```python
from build123d import *

# Parameters (mm, degrees)
BOSS_EXTRUDE1_DEPTH     = 11.5
SKETCH2_R               = 1.5
CUT_EXTRUDE1_DEPTH      = 1
CUT_EXTRUDE1_DEPTH_BACK = 15.4
FILLET1_R               = 1
FILLET2_R               = 1
FILLET3_R               = 1


with BuildPart() as part:
    # Sketch1 → Boss-Extrude1 (new body, symmetric)
    with BuildSketch(Plane.XY):
        Polygon((-5.2, 1), (5.2, 1), (5.2, 13.5), (7.2, 13.5), (7.2, -1), (-7.2, -1), (-7.2, 13.5), (-5.2, 13.5), align=None)
    extrude(amount=BOSS_EXTRUDE1_DEPTH, both=True)

    # Sketch2 → Cut-Extrude1 (cut, two sides)
    with BuildSketch(Plane(origin=(7.2, 0, 0), x_dir=(0, 0, -1), z_dir=(1, 0, 0))) as cut_extrude1_sk:
        with Locations((-7, 9)):
            Circle(SKETCH2_R)
        with Locations((7, 9)):
            Circle(SKETCH2_R)
    extrude(amount=CUT_EXTRUDE1_DEPTH, mode=Mode.SUBTRACT)
    extrude(cut_extrude1_sk.sketch, amount=-CUT_EXTRUDE1_DEPTH_BACK, mode=Mode.SUBTRACT)

    # Fillet1
    fillet1_edges = [part.edges().sort_by_distance(p)[0] for p in [
        (0, -1, -11.5),
        (0, -1, 11.5),
    ]]
    fillet(fillet1_edges, radius=FILLET1_R)

    # Fillet2
    fillet2_edges = [part.edges().sort_by_distance(p)[0] for p in [
        (-5.2, 1, 0),
        (5.2, 1, 0),
    ]]
    fillet(fillet2_edges, radius=FILLET2_R)

    # Fillet3
    fillet3_edges = [part.edges().sort_by_distance(p)[0] for p in [
        (-6.2, 13.5, -11.5),
        (6.2, 13.5, 11.5),
        (-6.2, 13.5, 11.5),
        (6.2, 13.5, -11.5),
    ]]
    fillet(fillet3_edges, radius=FILLET3_R)


solid = part.part
```
CAD build for the part. Positions are in the model's coordinates, mm. Coordinates: 2 decimals unless noted, no trailing zeros. Loops run counter-clockwise (first coordinate to the right, second up) from the corner with the lowest first, then second, coordinate; pieces in that order, holes last. Notation, with made-up numbers: (0, 48) - (29, 48) arc R10 cw to (29, 56) - close; hole circle Ø1 at (-33.5, -0.5). An arc over 180 degrees is marked (long way). Use CSV: the item, a comma, the result in double quotes. Start each with the question number.
Q1. Probe probe 1 along X at (y, z) = (9.5, 4); probe 2 along Y at (x, z) = (6.45, -7); probe 3 along Y at (x, z) = (-2, -6.5). List the from-to ranges inside material, lowest first. Write a range as from..to.
Q2. Two-plate mould, pull along X, no slides. Class faces 1 (the cylindrical face through (-0.101, -0.699, -11.215)), 2 (the flat face through (0, 1, 0)), 3 (the flat face through (7.2, 6, 0)), 4 (the cylindrical face through (4.915, 1.301, -0.161)): +X half, -X half, draft (parallel to the pull), parting line (faces both ways), or undercut.
Q3. Drop flat-ended pins along their axis: P1, Ø2, axis at x = -2, z = -9, coming from the +Y side; P2, Ø2.5, axis at y = 9, z = -7, coming from the -X side. Give the stop position or say it passes through.
Q4. Cut at B-B, the plane z = -7. List the corners of the cut face in (x, y).
Q5. Cut at A-A, the plane y = 9. List the corners of the cut face in (x, z), then the cut area to 3 significant figures.
Q6. Cut at D-D, the plane x = 5.5. List the corners of the cut face in (y, z).
Q7. Cut at C-C, the plane y = 11. List the corners of the cut face in (x, z), then the cut area to 3 significant figures.
Here are the results:
1,probe 1,"-7.2..-5.2, 5.2..7.2"
1,probe 2,"-1..7.5, 10.5..13.5"
1,probe 3,"-1..1"
2,face 1,"draft"
2,face 2,"undercut"
2,face 3,"+X half"
2,face 4,"undercut"
3,P1,"y = 1"
3,P2,"through"
4,outline,"(-7.2, -1) - (7.2, -1) - (7.2, 7.5) - (5.2, 7.5) - (5.2, 2) arc R1 cw to (4.2, 1) - (-4.2, 1) arc R1 cw to (-5.2, 2) - (-5.2, 7.5) - (-7.2, 7.5) - close; (-7.2, 10.5) - (-5.2, 10.5) - (-5.2, 13.5) - (-7.2, 13.5) - close; (5.2, 10.5) - (7.2, 10.5) - (7.2, 13.5) - (5.2, 13.5) - close"
5,outline,"(-7.2, -11.5) - (-5.2, -11.5) - (-5.2, -8.5) - (-7.2, -8.5) - close; (-7.2, -5.5) - (-5.2, -5.5) - (-5.2, 5.5) - (-7.2, 5.5) - close; (-7.2, 8.5) - (-5.2, 8.5) - (-5.2, 11.5) - (-7.2, 11.5) - close; (5.2, -11.5) - (7.2, -11.5) - (7.2, -8.5) - (5.2, -8.5) - close; (5.2, -5.5) - (7.2, -5.5) - (7.2, 5.5) - (5.2, 5.5) - close; (5.2, 8.5) - (7.2, 8.5) - (7.2, 11.5) - (5.2, 11.5) - close"
5,area,"68.0 mm2"
6,outline,"(-1, -10.5) arc R1 ccw to (0, -11.5) - (12.5, -11.5) arc R1 ccw to (13.5, -10.5) - (13.5, 10.5) arc R1 ccw to (12.5, 11.5) - (0, 11.5) arc R1 ccw to (-1, 10.5) - close; hole circle Ø3 at (9, -7); hole circle Ø3 at (9, 7)"
7,outline,"(-7.2, -11.5) - (-5.2, -11.5) - (-5.2, 11.5) - (-7.2, 11.5) - close; (5.2, -11.5) - (7.2, -11.5) - (7.2, 11.5) - (5.2, 11.5) - close"
7,area,"92.0 mm2"
